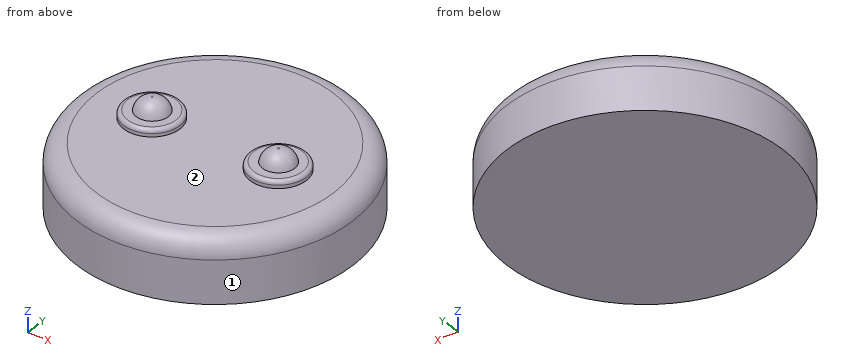
```python
from build123d import *

# Parameters (mm, degrees)
F0_R     = 4.3688
F1_DEPTH = 1.9812
F2_R     = 0.889
F3_DEPTH = 2.2098
F4_R     = 0.508
F5_DEPTH = 2.6162
F8_R     = 0.122642049
F9_R     = 0.6132102448


# Not quite as in the source:
# - a fillet or chamfer that OpenCascade refuses, or shapes differently, is made with other operations: its cross-section is extruded or revolved along the edge and cut away or added


with BuildPart() as f1:
    # F0 (on Top) → F1 (new body)
    with BuildSketch(Plane.XY):
        Circle(F0_R)
    extrude(amount=F1_DEPTH)

    # F2 (on Top) → F3 (join)
    with BuildSketch(Plane.XY):
        with Locations((-1.9812, 0)):
            Circle(F2_R)
        with Locations((1.9812, 0)):
            Circle(F2_R)
    extrude(amount=F3_DEPTH)

    # F4 (on Top) → F5 (join)
    with BuildSketch(Plane.XY):
        with Locations((-1.9675190561, 0)):
            Circle(F4_R)
        with Locations((1.9938375335, 0)):
            Circle(F4_R)
    extrude(amount=F5_DEPTH)

    # F6: fillet of radius 0.4905681959 on 1 edges, made by hand

    # F6_s1 → F6_t2 (revolve, cut)
    with BuildSketch(Plane.XZ):
        with BuildLine():
            ThreePointArc((-1.4595190561, 2.2098), (-1.6270859561, 2.5010964461), (-1.9428128276, 2.6162))
            Line((-1.9428128276, 2.6162), (-1.4595190561, 2.6162))
            Line((-1.4595190561, 2.6162), (-1.4595190561, 2.2098))
        make_face()
    revolve(axis=Axis((-1.9675190561, 0, 2.6162), (0, 0, 1)), mode=Mode.SUBTRACT)

    # F7: fillet of radius 0.4826 on 1 edges, made by hand

    # F7_s1 → F7_t2 (revolve, cut)
    with BuildSketch(Plane.XZ):
        with BuildLine():
            ThreePointArc((2.5018375335, 2.2098), (2.3384435237, 2.5008035403), (2.0252912923, 2.6162))
            Line((2.0252912923, 2.6162), (2.5018375335, 2.6162))
            Line((2.5018375335, 2.6162), (2.5018375335, 2.2098))
        make_face()
    revolve(axis=Axis((1.9938375335, 0, 2.6162), (0, 0, 1)), mode=Mode.SUBTRACT)

    # F8
    f8_edges = [f1.edges().sort_by_distance(p)[0] for p in [
        (-2.8702, 0, 2.2098),
        (1.0922, 0, 2.2098),
    ]]
    fillet(f8_edges, radius=F8_R)

    # F9
    f9_edges = [f1.edges().sort_by_distance(p)[0] for p in [
        (-4.3688, 0, 1.9812),
    ]]
    fillet(f9_edges, radius=F9_R)


solid = f1.part
```
Geometry check sheet. Reference: the model listing, model coordinates, mm. Face numbers are marked on the shaded views. A direction names the side the tool comes from. Round coordinates to 2 decimals unless told otherwise and drop trailing zeros. Order: outer loops, then holes, each group sorted by start corner. A loop starts at its lowest first (then second) coordinate and runs counter-clockwise, first axis right, second up. Notation, with made-up numbers: (27.5, 62.25) - (63.5, 62.25) arc R38 cw to (63.5, 100.25) - close; hole circle Ø4 at (87, -7.75). An arc over 180 degrees is marked (long way). Use a Markdown table: item, result. Add a question column.
(1) Material ranges on line 1 along Z through (x, y) = (1, 3); line 2 along X through (y, z) = (3.75, 0.55); line 3 along X through (y, z) = (-2.75, 0.45), recorded low to high. Write a range as [from, to].
(2) Tool access check on the marked faces 1 and 2. Record the directions out of +Z, -Z, +X, -X, +Y, -Y that give a thin tool (end or side, any length) a straight path to the whole face; none if there is none.
(3) Sectioned sample at B-B, the plane x = 0. Enter the section's corners in (y, z).
(4) Sectioned sample at A-A, the plane z = 0.65. Enter the section's corners in (x, y), and give its area (3 significant figures).
(5) Depth check by flat-ended pin: pin 1 (0.5 mm diameter, centred on x = 2, y = 0.5, fed in from +Z); pin 2 (1 mm diameter, centred on x = -2.5, z = 1.5, fed in from +Y). Enter the tip coordinate at first touch or a pass-through.
Answers below:
| question | item | result |
|---|---|---|
| 1 | line 1 | [0, 1.98] |
| 1 | line 2 | [-2.24, 2.24] |
| 1 | line 3 | [-3.39, 3.39] |
| 2 | face 1 | +Z, -Z |
| 2 | face 2 | +Z |
| 3 | outline | (-4.37, 0) - (4.37, 0) - (4.37, 1.37) arc R0.61 ccw to (3.76, 1.98) - (-3.76, 1.98) arc R0.61 ccw to (-4.37, 1.37) - close |
| 4 | outline | circle Ø8.74 at (0, 0) |
| 4 | area | 60.0 mm² |
| 5 | pin 1 | z = 2.56 |
| 5 | pin 2 | y = 3.88 |
